Geometry check sheet. Reference: the model listing, model coordinates, mm. Round coordinates to 2 decimals unless told otherwise and drop trailing zeros. Order: outer loops, then holes, each group sorted by start corner. A loop starts at its lowest first (then second) coordinate and runs counter-clockwise, first axis right, second up. Notation, with made-up numbers: (64.25, 40.25) - (85.25, 40.25) arc R33 ccw to (85.25, 71.25) - close; hole circle Ø2 at (-13, 53). An arc over 180 degrees is marked (long way). Return JSON: item names as keys, results as strings. Group by question number.
Q1. Sectioned sample at D-D, the plane x = -23. Record the cut outline in (y, z).
Q2. Sectioned sample at A-A, the plane y = 22.55. Record the cut outline in (x, z), then the cut area to 3 significant figures.
Q3. Material ranges on line 1 along Y through (x, z) = (-12.45, 1.1); line 2 along Y through (x, z) = (0, 1.8); line 3 along X through (y, z) = (-27.5, 0.6), recorded low to high.
Q4. Sectioned sample at C-C, the plane x = 0. Record the cut outline in (y, z), then the cut area to 3 significant figures.
Q5. Sectioned sample at B-B, the plane z = 2.5. Record the cut outline in (x, y).
```python
from build123d import *

# Parameters (mm, degrees)
F0_W     = 55
F0_H     = 65
F1_DEPTH = 3
F2_R     = 1.55
F3_DEPTH = 3
F4_R     = 8


with BuildPart() as f1:
    # F0 (on Top) → F1 (new body)
    with BuildSketch(Plane.XY):
        Rectangle(F0_W, F0_H)
    extrude(amount=F1_DEPTH)

    # F2 (on face) → F3 (cut, through all)
    with BuildSketch(Plane.XY.offset(3)):
        with Locations((-12.45, -14.95)):
            Circle(F2_R)
        with Locations((12.45, -14.95)):
            Circle(F2_R)
        with Locations((0, 22.55)):
            Circle(F2_R)
    extrude(amount=-F3_DEPTH, mode=Mode.SUBTRACT)

    # F4
    f4_edges = [f1.edges().sort_by_distance(p)[0] for p in [
        (27.5, -32.5, 1.5),
        (-27.5, -32.5, 1.5),
        (-27.5, 32.5, 1.5),
        (27.5, 32.5, 1.5),
    ]]
    fillet(f4_edges, radius=F4_R)


solid = f1.part
```
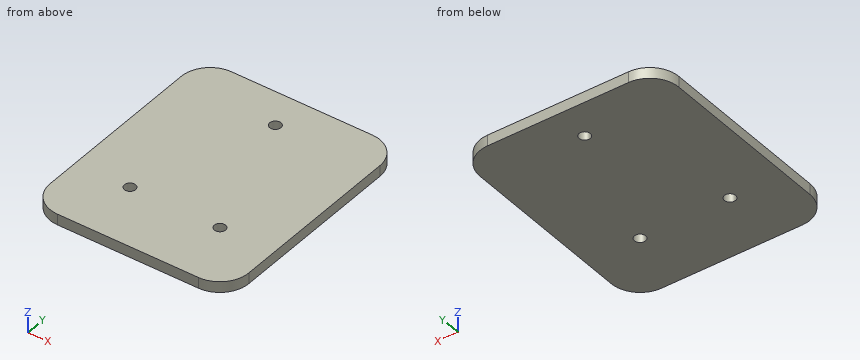
Reply:
{
 "1": {"outline": "(-31.69, 0) - (31.69, 0) - (31.69, 3) - (-31.69, 3) - close"},
 "2": {"outline": "(-27.5, 0) - (-1.55, 0) - (-1.55, 3) - (-27.5, 3) - close; (1.55, 0) - (27.5, 0) - (27.5, 3) - (1.55, 3) - close", "area": "156 mm^2"},
 "3": {"line 1": "-32.5 to -16.5, -13.4 to 32.5", "line 2": "-32.5 to 21, 24.1 to 32.5", "line 3": "-26.92 to 26.92"},
 "4": {"outline": "(-32.5, 0) - (21, 0) - (21, 3) - (-32.5, 3) - close; (24.1, 0) - (32.5, 0) - (32.5, 3) - (24.1, 3) - close", "area": "186 mm^2"},
 "5": {"outline": "(-27.5, -24.5) arc R8 ccw to (-19.5, -32.5) - (19.5, -32.5) arc R8 ccw to (27.5, -24.5) - (27.5, 24.5) arc R8 ccw to (19.5, 32.5) - (-19.5, 32.5) arc R8 ccw to (-27.5, 24.5) - close; hole circle Ø3.1 at (-12.45, -14.95); hole circle Ø3.1 at (0, 22.55); hole circle Ø3.1 at (12.45, -14.95)"}
}
